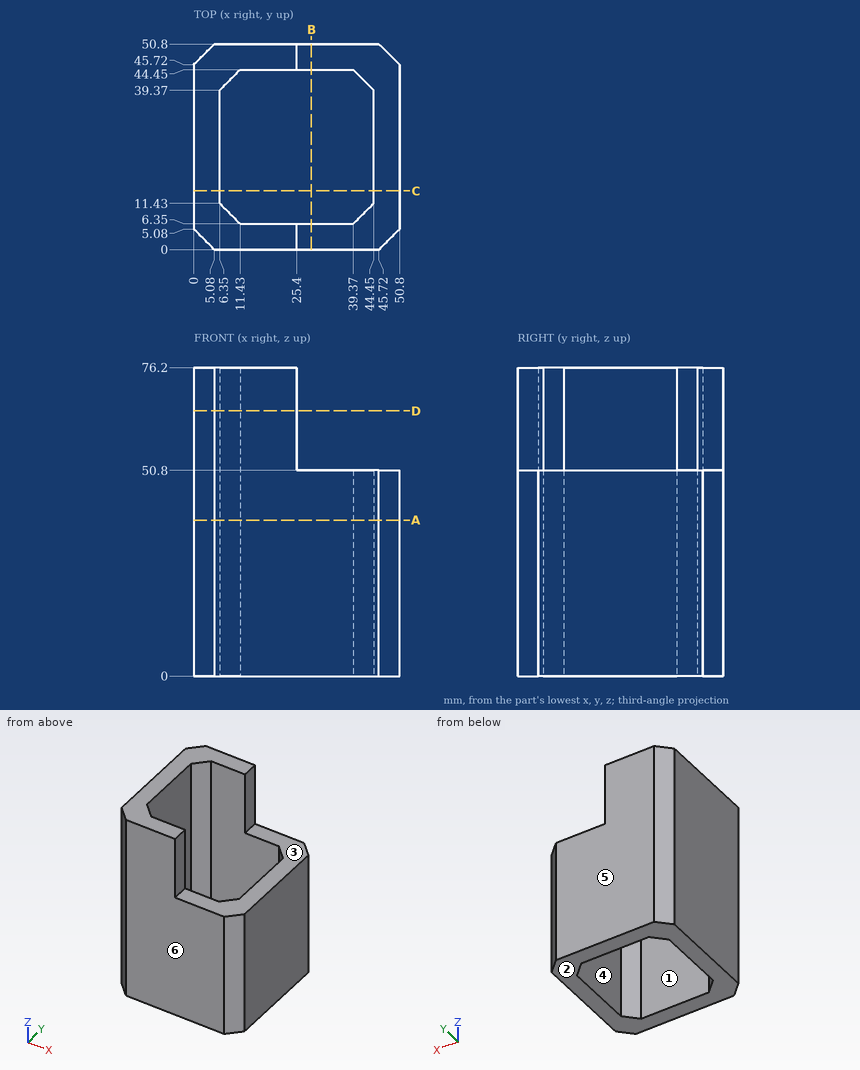
Could you check a few things on this drawing? It's one solid part, dimensions in mm from its lowest x, y, z. A direction names the side the tool comes from. Round coordinates to 2 decimals unless told otherwise and drop trailing zeros. Order: outer loops, then holes, each group sorted by start corner. A loop starts at its lowest first (then second) coordinate and runs counter-clockwise, first axis right, second up. Notation, with made-up numbers: M 62.5,36.5 L 95.5,36.5 A28 ccw 95.5,69.5 Z; hole C 87.5,47.25 d1. An arc over 180 degrees is marked long. Use a Markdown table: item, result.
1) If we mould it in two halves opening along Y, with no side actions, what happens to the marked faces 4, 5 and 6? For each: +Y half, -Y half, draft (parallel to the pull), parting line (faces both ways), or undercut.
Geometry says:
| item | result |
|---|---|
| face 4 | undercut |
| face 5 | +Y half |
| face 6 | -Y half |
2) Imagine slicing it at D-D (z = 65.5). List the corners of the cut face in (x, y) for me, then the cut area to 3 significant figures.
Geometry says:
| item | result |
|---|---|
| outline | M 0,5.08 L 5.08,0 L 25.4,0 L 25.4,6.35 L 11.43,6.35 L 6.35,11.43 L 6.35,39.37 L 11.43,44.45 L 25.4,44.45 L 25.4,50.8 L 5.08,50.8 L 0,45.72 Z |
| area | 565 mm² |
3) Imagine slicing it at A-A (z = 38.5). List the corners of the cut face in (x, y) for me.
Geometry says:
| item | result |
|---|---|
| outline | M 0,5.08 L 5.08,0 L 45.72,0 L 50.8,5.08 L 50.8,45.72 L 45.72,50.8 L 5.08,50.8 L 0,45.72 Z; hole M 6.35,11.43 L 11.43,6.35 L 39.37,6.35 L 44.45,11.43 L 44.45,39.37 L 39.37,44.45 L 11.43,44.45 L 6.35,39.37 Z |
4) Imagine slicing it at B-B (x = 29). List the corners of the cut face in (y, z) for me, then the cut area to 3 significant figures.
Geometry says:
| item | result |
|---|---|
| outline | M 0,0 L 6.35,0 L 6.35,50.8 L 0,50.8 Z; M 44.45,0 L 50.8,0 L 50.8,50.8 L 44.45,50.8 Z |
| area | 645 mm² |
5) If I drill on line 1 along Y through (x, z) = (15, 39.5); line 2 along Z through (x, y) = (36, 4.5), over which ranges is the centre line in solid material (lowest first)?
Geometry says:
| item | result |
|---|---|
| line 1 | y = 0 to 6.35, 44.45 to 50.8 |
| line 2 | z = 0 to 50.8 |
6) I'm going to push flat-ended pins straight in: P1, Ø7.5, axis at x = 44, y = 13.5, coming from the +Z side; P2, Ø7, axis at y = 48.5, z = 66, coming from the +X side. Where does each tip first touch, or does it pass through?
Geometry says:
| item | result |
|---|---|
| P1 | stops at z = 50.8 |
| P2 | stops at x = 25.4 |
7) On a 3-axis mill with a long thin cutter (end or side, diameter ignored), from which of +Z, -Z, +X, -X, +Y, -Y can I reach the whole of each face in a straight line? I mean the marked faces 1, 2 and 3. Say none if no direction works.
Geometry says:
| item | result |
|---|---|
| face 1 | +Z, -Z |
| face 2 | -Z, +X, -X, +Y, -Y |
| face 3 | +Z, +X, +Y, -Y |
8) Imagine slicing it at C-C (y = 14.5). List the corners of the cut face in (x, z) for me.
Geometry says:
| item | result |
|---|---|
| outline | M 0,0 L 6.35,0 L 6.35,76.2 L 0,76.2 Z; M 44.45,0 L 50.8,0 L 50.8,50.8 L 44.45,50.8 Z |
